from build123d import *

# Parameters (mm, degrees)
F2_DEPTH      = 150
F2_DEPTH_BACK = 150


with BuildPart() as f2:
    # F1 (on Front) → F2 (new body, two sides)
    with BuildSketch(Plane.XZ) as f2_sk:
        Polygon((-170, 0), (-150, 0), (-150, 18), (-170, 18), (-170, 15), (-153, 15), (-153, 3), (-170, 3), align=None)
    extrude(amount=F2_DEPTH)
    extrude(f2_sk.sketch, amount=-F2_DEPTH_BACK)


solid = f2.part
Could you check a few things on this model? Use its own coordinates, in mm. A direction names the side the tool comes from. Round coordinates to 2 decimals unless told otherwise and drop trailing zeros. Write each loop counter-clockwise with the first axis right and the second up, starting at its lowest first coordinate (ties: lowest second). Pieces come first, ordered by that corner, then holes. Notation, with made-up numbers: (47.25, 46.5) - (68.25, 46.5) arc R35 ccw to (68.25, 82.5) - close; hole circle Ø2 at (-24.75, -6). An arc over 180 degrees is marked (long way). Use a Markdown table: item, result.
Q1. I want a section at A-A (x = -164.5). List the corners of the cut face in (y, z) for me.
Output values:
| item | result |
|---|---|
| outline | (-150, 0) - (150, 0) - (150, 3) - (-150, 3) - close; (-150, 15) - (150, 15) - (150, 18) - (-150, 18) - close |
Q2. I want a section at C-C (z = 10). List the corners of the cut face in (x, y) for me.
Output values:
| item | result |
|---|---|
| outline | (-153, -150) - (-150, -150) - (-150, 150) - (-153, 150) - close |
Q3. For faces 1 (the flat face through (-150, -2, 9)), 2 (the flat face through (-162, -2, 15)), which set-ups out of +Z, -Z, +X, -X, +Y, -Y let a thin tool reach every point of the face, with its end or its side?
Output values:
| item | result |
|---|---|
| face 1 | +Z, -Z, +X, +Y, -Y |
| face 2 | -X, +Y, -Y |
Q4. For pin 1 (6 mm diameter, centred on x = -158, z = 13, fed in from +Y), with a flat end and sliding along its axis, tell me the tip position at first contact or that it passes through.
Output values:
| item | result |
|---|---|
| pin 1 | y = 150 |
Q5. Thinking about a two-plate mould opening in Z: for faces 3 (the flat face through (-153, -2, 9)), 4 (the flat face through (-161, -2, 3)), 5 (the flat face through (-158, -150, 17)), 6 (the flat face through (-160, -2, 0)), which applies, released by +Z, released by -Z, zero draft, split by the parting line, or undercut?
Output values:
| item | result |
|---|---|
| face 3 | undercut |
| face 4 | undercut |
| face 5 | zero draft |
| face 6 | released by -Z |
Q6. I want a section at B-B (y = 57). List the corners of the cut face in (x, z) for me.
Output values:
| item | result |
|---|---|
| outline | (-170, 0) - (-150, 0) - (-150, 18) - (-170, 18) - (-170, 15) - (-153, 15) - (-153, 3) - (-170, 3) - close |
Q7. Please list where these lines run through material, in increasing order: L1, parallel to Z at x = -166, y = 130; L2, parallel to X at y = -109, z = 5.
Output values:
| item | result |
|---|---|
| L1 | 0 to 3, 15 to 18 |
| L2 | -153 to -150 |
